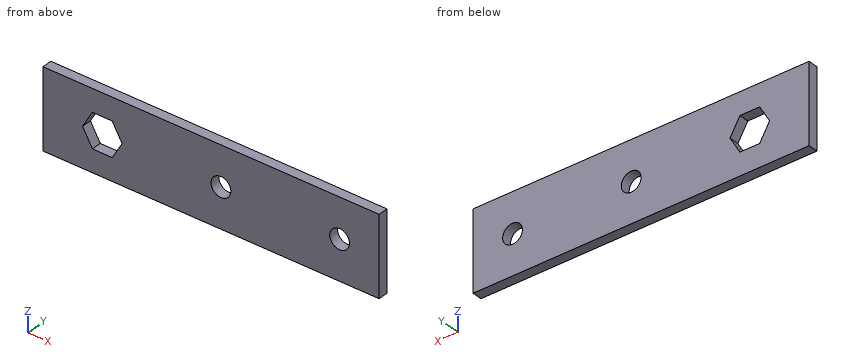
Autodesk Inventor part; units mm, degrees
ref_plane "YZ Plane" through (0, 0, 0) normal (1, 0, 0) x (0, 1, 0)
ref_plane "XZ Plane" through (0, 0, 0) normal (0, 1, 0) x (-1, 0, 0)
ref_plane "XY Plane" through (0, 0, 0) normal (0, 0, 1) x (1, 0, 0)
sketch "Sketch1" plane through (0, 0, 0) normal (0, 1, 0) x (-1, 0, 0)
  line L0 (50.8, 12.7) -> (-50.8, 12.7)
  line L1 (-50.8, 12.7) -> (-50.8, -12.7)
  line L2 (-50.8, -12.7) -> (50.8, -12.7)
  line L3 (50.8, -12.7) -> (50.8, 12.7)
  line L4 (50.8, 12.7) -> (-50.8, -12.7) construction
  line L5 (-50.8, 12.7) -> (50.8, -12.7) construction
  point P0 (0, 0)
  dimension "d0" = 101.6
  dimension "d1" = 25.4
extrude "Extrusion1" add sketch "Sketch1" along normal blind 3.175
sketch "Sketch2" plane through (0, 3.175, 0) normal (0, 1, 0) x (1, 0, 0)
  line L0 (-50.8, 12.7) -> (-50.8, -12.7)
  circle A0 centre (0, 0) radius 6.35
  line L1 (0, 0) -> (0, 6.35)
  line L2 (0, 0) -> (6.35, 0)
  line L3 (6.35, 0) -> (3.175, -5.4993)
  line L4 (3.175, -5.4993) -> (-3.175, -5.4993)
  line L5 (-3.175, -5.4993) -> (-6.35, 0)
  line L6 (-6.35, 0) -> (-3.175, 5.4993)
  line L7 (-3.175, 5.4993) -> (3.175, 5.4993)
  line L8 (3.175, 5.4993) -> (6.35, 0)
  dimension "d4" = 12.7
extrude "Extrusion2" cut sketch "Sketch2" against normal blind 3.175 contours L3 L4 L5 L6 L7 L1 L2 | L2 L1 L7 L8
sketch "Sketch3" plane through (0, 3.175, 0) normal (0, 1, 0) x (1, 0, 0)
  line L0 (50.8, 12.7) -> (-50.8, 12.7)
  line L1 (-50.8, 12.7) -> (-50.8, -12.7)
  line L2 (0, 0) -> (-38.1, 0)
  line L3 (-38.1, 0) -> (38.1, 0)
  circle A0 centre (-38.1, 0) radius 3.175
  circle A1 centre (38.1, 0) radius 3.175
  dimension "d7" = 38.1
  dimension "d8" = 76.2
  dimension "d9" = 0
  dimension "d10" = 6.35
  dimension "d11" = 6.35
extrude "Extrusion3" cut sketch "Sketch3" against normal blind 3.175
sketch "Sketch4" plane through (0, 3.175, 0) normal (0, 1, 0) x (1, 0, 0)
  circle A0 centre (-38.1, 0) radius 3.175
  line L0 (-50.8, 12.7) -> (-12.7, 12.7)
  line L1 (-12.7, 12.7) -> (-12.7, -12.7)
  line L2 (-12.7, -12.7) -> (-50.8, -12.7)
  line L3 (-50.8, -12.7) -> (-50.8, 12.7)
  point P0 (0, 0)
  dimension "d14" = 38.1
  dimension "d15" = 25.4
extrude "Extrusion4" cut sketch "Sketch4" against normal blind 25.4
sketch "Sketch5" plane through (0, 3.175, 0) normal (0, 1, 0) x (1, 0, 0)
  circle A0 centre (38.1, 0) radius 3.175
  line L0 (3.175, -5.4993) -> (-3.175, -5.4993)
  line L1 (38.1, 0) -> (76.2, 0)
  line L2 (38.1, 0) -> (76.2, 0) construction
  circle A1 centre (76.2, 0) radius 3.175
  line L3 (50.8, 12.7) -> (88.9, 12.7)
  line L4 (88.9, 12.7) -> (88.9, -12.7)
  line L5 (88.9, -12.7) -> (50.8, -12.7)
  line L6 (50.8, -12.7) -> (50.8, 12.7)
  point P0 (0, 0)
  dimension "d18" = 38.1
  dimension "d19" = 0
  dimension "d20" = 6.35
  dimension "d21" = 38.1
  dimension "d22" = 25.4
extrude "Extrusion5" add sketch "Sketch5" against normal blind 3.175 contours L6 L3 L4 L5
sketch "Sketch6" plane through (-12.7, 3.175, -12.7) normal (-1, 0, 0) x (0, 0, 1)
  line L0 (25.4, -3.175) -> (0, -3.175)
  line L1 (25.4, 0) -> (25.4, -3.175)
  line L2 (0, 0) -> (25.4, 0)
  line L3 (0, -3.175) -> (0, 0)
  point P0 (12.7, -3.175)
extrude "Extrusion6" add sketch "Sketch6" along normal blind 6.35
properties part number "ArmBrace"
Read the model definition and answer for the solid it produces. Units are mm, in the model's axes. Give positions to 0.01 mm unless a question says otherwise; leave off trailing zeros. Loops run counter-clockwise (first coordinate to the right, second up) from the corner with the lowest first, then second, coordinate; pieces in that order, holes last. Notation, with made-up numbers: (9, 17.25) -> (57, 17.25) arc R20 cw to (57, 23.25) -> close; hole circle Ø6 at (35.25, 20). An arc over 180 degrees is marked (long way). Use a Markdown table: item, result.
Q1. Find the intervals of material crossed by line 1 along Z through (x, y) = (76.2, 0.65) (3 decimals); line 2 along X through (y, z) = (2, -0.5); line 3 along X through (y, z) = (1.5, 2.25), in increasing order.
Solved:
| item | result |
|---|---|
| line 1 | z = -12.7 to -3.175, 3.175 to 12.7 |
| line 2 | x = -19.05 to -6.06, 6.06 to 34.96, 41.24 to 73.06, 79.34 to 88.9 |
| line 3 | x = -19.05 to -5.05, 5.05 to 35.86, 40.34 to 73.96, 78.44 to 88.9 |
Q2. Section A-A, the plane x = 76.2 is taken. Determine the outline of the cut face in (y, z) (3 decimals), then the cut area to 3 significant figures.
Solved:
| item | result |
|---|---|
| outline | (0, -12.7) -> (3.175, -12.7) -> (3.175, -3.175) -> (0, -3.175) -> close; (0, 3.175) -> (3.175, 3.175) -> (3.175, 12.7) -> (0, 12.7) -> close |
| area | 60.5 mm^2 |
Q3. Section B-B, the plane y = 1.55 is taken. Determine the outline of the cut face in (x, z) (3 decimals), then the cut area to 3 significant figures.
Solved:
| item | result |
|---|---|
| outline | (-19.05, -12.7) -> (88.9, -12.7) -> (88.9, 12.7) -> (-19.05, 12.7) -> close; hole (-6.35, 0) -> (-3.175, -5.499) -> (3.175, -5.499) -> (6.35, 0) -> (3.175, 5.499) -> (-3.175, 5.499) -> close; hole circle Ø6.35 at (38.1, 0); hole circle Ø6.35 at (76.2, 0) |
| area | 2,570 mm^2 |
Q4. Section C-C, the plane z = -4.25 is taken. Determine the outline of the cut face in (x, y) (3 decimals).
Solved:
| item | result |
|---|---|
| outline | (-19.05, 0) -> (-3.896, 0) -> (-3.896, 3.175) -> (-19.05, 3.175) -> close; (3.896, 0) -> (88.9, 0) -> (88.9, 3.175) -> (3.896, 3.175) -> close |
